Autodesk Inventor part; units mm, degrees
ref_plane "YZ Plane" through (0, 0, 0) normal (1, 0, 0) x (0, 1, 0)
ref_plane "XZ Plane" through (0, 0, 0) normal (0, 1, 0) x (-1, 0, 0)
ref_plane "XY Plane" through (0, 0, 0) normal (0, 0, 1) x (1, 0, 0)
sketch "Skizze1" plane through (0, 0, 0) normal (0, 1, 0) x (-1, 0, 0)
  line L0 (3.5, -2.0207) -> (0, -4.0415)
  line L1 (0, -4.0415) -> (-3.5, -2.0207)
  line L2 (-3.5, -2.0207) -> (-3.5, 2.0207)
  line L3 (-3.5, 2.0207) -> (0, 4.0415)
  line L4 (0, 4.0415) -> (3.5, 2.0207)
  line L5 (3.5, 2.0207) -> (3.5, -2.0207)
  point P0 (0, 0)
  point P1 (0, 0)
  dimension "d0" = 7
extrude "Extrusion1" add sketch "Skizze1" along normal blind 45
sketch "Skizze2" plane through (0, 45, 0) normal (0, 1, 0) x (1, 0, 0)
  point P0 (0, 0)
  point P1 (0, 0)
hole "Bohrung1" at (0, 45, 0) direction (0, -1, 0) diameter 3.242 depth 11.8 tip angle 118
sketch "Skizze3" plane through (0, 0, 0) normal (0, -1, 0) x (1, 0, 0)
  point P0 (0, 0)
  point P1 (0, 0)
hole "Bohrung2" at (0, 0, 0) direction (0, 1, 0) diameter 3.242 depth 11.8 tip angle 118
chamfer "Fasen1" distance 0.5 angle 45 12 edges at (-1.75, 45, 3.0311) (1.75, 45, 3.0311) (3.5, 45, 0) (1.75, 45, -3.0311) (-1.75, 45, -3.0311) (-3.5, 45, 0) (-3.5, 0, 0) (-1.75, 0, 3.0311) (1.75, 0, 3.0311) (3.5, 0, 0) (1.75, 0, -3.0311) (-1.75, 0, -3.0311)
properties part number "Abstandsbolzen 45mm" material "Aluminium 6061"
For this review, take the finished solid that the model builds, in its own axes (mm). A direction names the side the tool comes from. Round coordinates to 2 decimals unless told otherwise and drop trailing zeros. Write each loop counter-clockwise with the first axis right and the second up, starting at its lowest first coordinate (ties: lowest second). Pieces come first, ordered by that corner, then holes. Notation, with made-up numbers: (73.5, 10) - (82.5, 10) arc R27 ccw to (82.5, 32) - close; hole circle Ø1 at (-25.75, 35). An arc over 180 degrees is marked (long way). Put each result on its own line as item: value.
Q1. We need section A-A (y = 35). Give the boundary of the cut face in (x, z), and give its area (3 significant figures).
Solved:
outline: (-3.5, -2.02) - (0, -4.04) - (3.5, -2.02) - (3.5, 2.02) - (0, 4.04) - (-3.5, 2.02) - close; hole circle Ø3.24 at (0, 0)
area: 34.2 mm2
Q2. We need section B-B (z = -3). Give the boundary of the cut face in (x, y), and give its area (3 significant figures).
Solved:
outline: (-1.8, 0.5) - (-0.8, 0) - (0.8, 0) - (1.8, 0.5) - (1.8, 44.5) - (0.8, 45) - (-0.8, 45) - (-1.8, 44.5) - close
area: 161 mm2
Q3. Insertion check: pin 1 Ø1.5 at (x, y) = (2.5, 20) entering from +Z; pin 2 Ø1 at (x, y) = (-1, 25.5) entering from +Z; pin 3 Ø3 at (x, z) = (0, 0) entering from -Y. Each pin has a flat end and moves straight along its axis. Give the tip position at first contact, or say it passes through.
Solved:
pin 1: stops at z = 3.03
pin 2: stops at z = 3.75
pin 3: stops at y = 11.87
Q4. Machinability: for faces 1 (the face through (1.438, 5.983, -0.748)), 2 (the face through (-1.6, 44.75, -2.83)), which of the approach directions +Z, -Z, +X, -X, +Y, -Y give a long, thin tool a straight path to every point of the face, cutting with its end or side? Answer none if there is none.
Solved:
face 1: -Y
face 2: -Z, -X, +Y
Q5. Mouldability with a two-part tool opening along Z and no side actions: class faces 3 (the face through (1.438, 39.017, 0.748)), 4 (the face through (0.19, 32.395, -0.207)), 5 (the face through (-3.5, 22, 0)), 6 (the face through (-1.6, 44.75, 2.83)) as released by +Z, released by -Z, zero draft, split by the parting line, or undercut.
Solved:
face 3: undercut
face 4: undercut
face 5: zero draft
face 6: released by +Z
Q6. Wall thickness on probe 1 along Z at (x, y) = (0, 6); probe 2 along X at (y, z) = (5.25, 0); probe 3 along Z at (x, y) = (-1, 8): over which ranges is each line inside the solid? List them lowest first.
Solved:
probe 1: z = -4.04 to -1.62, 1.62 to 4.04
probe 2: x = -3.5 to -1.62, 1.62 to 3.5
probe 3: z = -3.46 to -1.28, 1.28 to 3.46
Q7. We need section C-C (y = 18.5). Give the boundary of the cut face in (x, z), and give its area (3 significant figures).
Solved:
outline: (-3.5, -2.02) - (0, -4.04) - (3.5, -2.02) - (3.5, 2.02) - (0, 4.04) - (-3.5, 2.02) - close
area: 42.4 mm2
